For this review, take the finished solid that the model builds, in its own axes (mm). Give positions to 0.01 mm unless a question says otherwise; leave off trailing zeros. Order: outer loops, then holes, each group sorted by start corner. A loop starts at its lowest first (then second) coordinate and runs counter-clockwise, first axis right, second up. Notation, with made-up numbers: (45.25, -32.75) - (70.25, -32.75) arc R18 cw to (70.25, -21.75) - close; hole circle Ø6 at (-19, 87.25). An arc over 180 degrees is marked (long way). One line per item, written item: value.
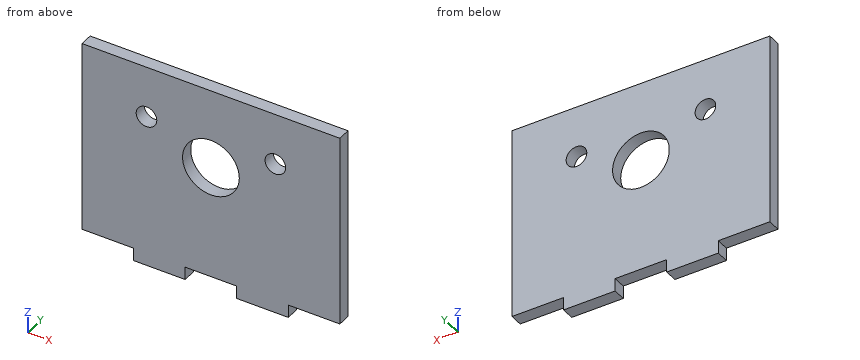
```python
from build123d import *

# Parameters (mm, degrees)
SKETCH1_R           = 4
BOSS_EXTRUDE1_DEPTH = 5
CUT_EXTRUDE1_REACH  = 7
SKETCH2_R           = 11


with BuildPart() as part:
    # Sketch1 → Boss-Extrude1 (new body)
    with BuildSketch(Plane(origin=(0, 0, 0), x_dir=(1, 0, 0), z_dir=(0, 1, 0))):
        Polygon((-50, 44), (-30, 44), (-30, 49), (-10, 49), (-10, 44), (10, 44), (10, 49), (30, 49), (30, 44), (50, 44), (50, -31), (-50, -31), align=None)
        Circle(SKETCH1_R, mode=Mode.SUBTRACT)
        with Locations((25, -11)):
            Circle(SKETCH1_R, mode=Mode.SUBTRACT)
        with Locations((-25, -11)):
            Circle(SKETCH1_R, mode=Mode.SUBTRACT)
    extrude(amount=BOSS_EXTRUDE1_DEPTH)

    # Sketch2 → Cut-Extrude1 (cut, up to next)
    with BuildSketch(Plane(origin=(0, 5, 0), x_dir=(1, 0, 0), z_dir=(0, 1, 0)), mode=Mode.PRIVATE) as cut_extrude1_sk1:
        Circle(SKETCH2_R)
    cut_extrude1_tool1 = extrude(cut_extrude1_sk1.sketch, amount=-CUT_EXTRUDE1_REACH, mode=Mode.PRIVATE) & part.part
    add(cut_extrude1_tool1.solids().sort_by_distance((0, 5, 0))[0], mode=Mode.SUBTRACT)


solid = part.part
```
(1) Take a section at C-C (y = 1.45). Write out the cut boundary in (x, z).
Answers below:
outline: (-50, -44) - (-30, -44) - (-30, -49) - (-10, -49) - (-10, -44) - (10, -44) - (10, -49) - (30, -49) - (30, -44) - (50, -44) - (50, 31) - (-50, 31) - close; hole circle Ø8 at (-25, 11); hole circle Ø22 at (0, 0); hole circle Ø8 at (25, 11)
(2) Take a section at A-A (z = 0). Write out the cut boundary in (x, y), then the cut area to 3 significant figures.
Answers below:
outline: (-50, 0) - (-11, 0) - (-11, 5) - (-50, 5) - close; (11, 0) - (50, 0) - (50, 5) - (11, 5) - close
area: 390 mm^2
(3) Take a section at D-D (x = 37). Write out the cut boundary in (y, z).
Answers below:
outline: (0, -44) - (5, -44) - (5, 31) - (0, 31) - close
(4) For P1, Ø2.5, axis at x = -36.5, y = 1.5, coming from the -Z side; P2, Ø2.5, axis at y = 2, z = -46, coming from the -X side; P3, Ø2, axis at x = -40, z = -4, coming from the -Y side; P4, Ø1.5, axis at y = 2.5, z = -47.5, coming from the +X side, all flat-tipped, find the tip position at first contact; note any pin that passes through.
Answers below:
P1: stops at z = -44
P2: stops at x = -30
P3: stops at y = 0
P4: stops at x = 30
(5) Take a section at B-B (x = 25). Write out the cut boundary in (y, z).
Answers below:
outline: (0, -49) - (5, -49) - (5, 7) - (0, 7) - close; (0, 15) - (5, 15) - (5, 31) - (0, 31) - close
(6) Wall thickness on line 1 (Z direction, x = -25, y = 3.05); line 2 (X direction, y = 3.25, z = 0); line 3 (Z direction, x = 0, y = 2.25): over which ranges is each line inside the solid? List them lowest first. Write a range as from..to.
Answers below:
line 1: z = -49..7, 15..31
line 2: x = -50..-11, 11..50
line 3: z = -44..-11, 11..31
